Geometry: final body of the model. Coordinates: model frame, mm. A direction names the side the tool comes from. Coordinates: 2 decimals unless noted, no trailing zeros. Order: outer loops, then holes, each group sorted by start corner. A loop starts at its lowest first (then second) coordinate and runs counter-clockwise, first axis right, second up. Notation, with made-up numbers: (47.25, 21.5) -> (96.25, 21.5) arc R20 cw to (96.25, 34.5) -> close; hole circle Ø7 at (54, 58.5). An arc over 180 degrees is marked (long way). Answer in a Markdown table with one row per item. Add a question column.
1) Ray query, line 1 (X direction, y = 20, z = -2.5); line 2 (Y direction, x = 13, z = -12). Return the intervals inside material, ascending. Write a range as from..to.
2) Set-up query: faces 4 (the face through (-16, 25.4, 0)), 5 (the face through (0, 13, 13.2)). Return all of +Z, -Z, +X, -X, +Y, -Y with unobstructed straight access to the full face (end or side cutting, diameter ignored); none if empty.
3) Pull-direction query (X, two-part tool) for faces 1 (the face through (13.2, 13, 0)), 2 (the face through (0, -5, 0)), 3 (the face through (18.2, 10, 0)); classes: +X half, -X half, draft (parallel to the pull), parting line (faces both ways), or undercut.
4) Contact query for a flat-ended pin moving along its axis: P1, Ø21, axis at x = -2, z = -1.5, coming from the +Y side. Output: stop coordinate, or through.
5) Section query C-C on x = -8. Return the cut outline in (y, z), then the cut area to 3 significant figures.
6) Section query B-B on z = 5.5. Return the cut outline in (x, y).
7) Section query A-A on y = 5.5. Return the cut outline in (x, z), then the cut area to 3 significant figures.
Autodesk Fusion 360 part; units mm, degrees
sketch "Sketch1" plane through (0, 0, 0) normal (0, 1, 0) x (1, 0, 0)
  line L0 (18.2, 18.2) -> (-18.2, 18.2)
  line L1 (-18.2, 18.2) -> (-18.2, -18.2)
  line L2 (-18.2, -18.2) -> (18.2, -18.2)
  line L3 (18.2, -18.2) -> (18.2, 18.2)
  line L4 (18.2, 18.2) -> (-18.2, -18.2) construction
  line L5 (-18.2, 18.2) -> (18.2, -18.2) construction
  line L6 (-18.2, 18.2) -> (18.2, 18.2)
  line L7 (18.2, 18.2) -> (18.2, 13.2)
  line L8 (18.2, 13.2) -> (-18.2, 13.2)
  line L9 (-18.2, 13.2) -> (-18.2, 18.2)
  line L10 (18.2, -18.2) -> (-18.2, -18.2)
  line L11 (-18.2, -18.2) -> (-18.2, -13.2)
  line L12 (-18.2, -13.2) -> (18.2, -13.2)
  line L13 (18.2, -13.2) -> (18.2, -18.2)
  line L14 (-18.2, 13.2) -> (-13.2, 13.2)
  line L15 (-13.2, 13.2) -> (-13.2, -13.2)
  line L16 (-13.2, -13.2) -> (-18.2, -13.2)
  line L17 (-18.2, -13.2) -> (-18.2, 13.2)
  line L18 (18.2, 13.2) -> (13.2, 13.2)
  line L19 (13.2, 13.2) -> (13.2, -13.2)
  line L20 (13.2, -13.2) -> (18.2, -13.2)
  line L21 (18.2, -13.2) -> (18.2, 13.2)
  dimension "d4" = 36.4
  dimension "d5" = 36.4
  dimension "d6" = 5
  dimension "d7" = 5
  dimension "d8" = 5
  dimension "d9" = 5
extrude "Extrude1" add sketch "Sketch1" along normal blind 25.4 contours L0 L1 L3 L6 L7 L8 L9 L14 L18 | L3 L8 L12 L18 L19 L20 L21 | L1 L8 L12 L14 L15 L16 L17 | L1 L2 L3 L10 L11 L12 L13 L16 L20
extrude "Extrude2" add 1 faces at (-16.5333, 0, 4.4) along direction (0, -1, 0) blind 5
extrude "Extrude3" add sketch "Sketch1" against normal blind 5 contours L8 L12 L15 L19
equation "ONEINCH = 25.4 mm"
equation "TOLERANCE = 0.5 mm"
equation "WALL_THICKNESS = 5 mm"
equation "d4 = ONEINCH + ( 2 * TOLERANCE ) + ( WALL_THICKNESS * 2 )"
equation "d5 = ONEINCH + ( 2 * TOLERANCE ) + ( WALL_THICKNESS * 2 )"
equation "d6 = WALL_THICKNESS"
equation "d7 = WALL_THICKNESS"
equation "d8 = WALL_THICKNESS"
equation "d9 = WALL_THICKNESS"
equation "d10 = ONEINCH"
equation "d12 = WALL_THICKNESS"
Result:
| question | item | result |
|---|---|---|
| 1 | line 1 | -18.2..-13.2, 13.2..18.2 |
| 1 | line 2 | -5..0 |
| 2 | face 4 | +Z, -Z, +X, -X, +Y |
| 2 | face 5 | +Y |
| 3 | face 1 | undercut |
| 3 | face 2 | draft |
| 3 | face 3 | +X half |
| 4 | P1 | y = 0 |
| 5 | outline | (-5, -18.2) -> (25.4, -18.2) -> (25.4, -13.2) -> (0, -13.2) -> (0, 13.2) -> (25.4, 13.2) -> (25.4, 18.2) -> (-5, 18.2) -> close |
| 5 | area | 436 mm2 |
| 6 | outline | (-18.2, -5) -> (18.2, -5) -> (18.2, 25.4) -> (13.2, 25.4) -> (13.2, 0) -> (-13.2, 0) -> (-13.2, 25.4) -> (-18.2, 25.4) -> close |
| 7 | outline | (-18.2, -18.2) -> (18.2, -18.2) -> (18.2, 18.2) -> (-18.2, 18.2) -> close; hole (-13.2, -13.2) -> (13.2, -13.2) -> (13.2, 13.2) -> (-13.2, 13.2) -> close |
| 7 | area | 628 mm2 |
